Part model, mm, in its own coordinate system. Face numbers are marked on the shaded views. Give positions to 0.01 mm unless a question says otherwise; leave off trailing zeros. Write each loop counter-clockwise with the first axis right and the second up, starting at its lowest first coordinate (ties: lowest second). Pieces come first, ordered by that corner, then holes. Notation, with made-up numbers: M 43,88 L 66,88 A30 cw 66,120 Z; hole C 55,-23 d6. An arc over 180 degrees is marked long. Use a Markdown table: item, result.
```python
from build123d import *

# Parameters (mm, degrees)
F2_R = 1.49999


# Not quite as in the source:
# - a fillet or chamfer is up to 0.001 mm smaller than in the source, because OpenCascade refuses the exact size


with BuildPart() as f1:
    # F0 (on Right) → F1 (revolve)
    with BuildSketch(Plane.YZ):
        Polygon((43, 3), (43, 0), (60, 0), (69.0046720892, 153), (73.5, 153), (73.5, 156), (71, 156), (71, 170), (67, 170), (57.1713709877, 3), (46, 3), (46, 6), (0, 6), (0, 3), align=None)
    revolve(axis=Axis((0, 0, 4.5), (0, 0, -1)))

    # F2 (radius 1.5 in the source; OpenCascade refuses exactly that, so slightly less here)
    f2_edges = [f1.edges().sort_by_distance(p)[0] for p in [
        (0, -43, 0),
        (0, -60, 0),
        (0, -43, 3),
    ]]
    fillet(f2_edges, radius=F2_R)


solid = f1.part
```
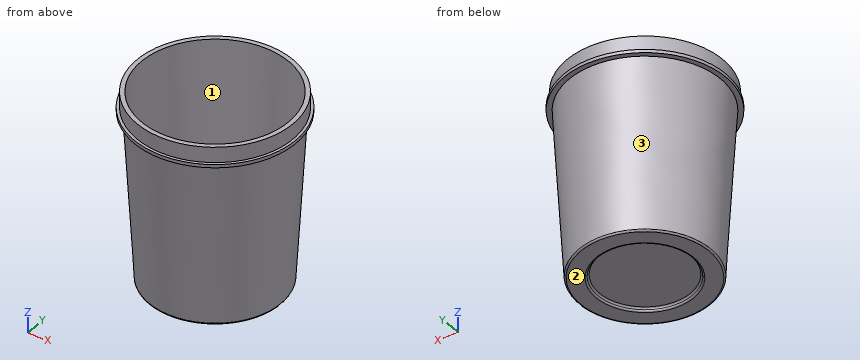
1. Cut at D-D, the plane z = 74. Give the cut face in (x, y), then the cut area to 3 significant figures.
Findings below:
| item | result |
|---|---|
| outline | C 0,0 d128.71; hole C 0,0 d122.7 |
| area | 1,190 mm2 |
2. Drop flat-ended pins along their axis: P1, Ø1.5, axis at x = -36.5, z = 97.5, coming from the +Y side; P2, Ø1, axis at x = -47.5, y = -4.5, coming from the +Z side; P3, Ø4, axis at x = -41.5, z = 137, coming from the +Y side. Give the stop position or say it passes through.
Findings below:
| item | result |
|---|---|
| P1 | y = 55.17 |
| P2 | z = 3 |
| P3 | y = 55.44 |
3. Drill centre lines: L1, parallel to X at y = 0, z = 1.55; L2, parallel to X at y = -33.5, z = 16; L3, parallel to Z at x = -11.5, y = -3. Where is each one in solid material? Low to high.
Findings below:
| item | result |
|---|---|
| L1 | -60.09 to -43, 43 to 60.09 |
| L2 | -50.91 to -47.27, 47.27 to 50.91 |
| L3 | 3 to 6 |
4. Cut at C-C, the plane z = 115. Give the cut face in (x, y), then the cut area to 3 significant figures.
Findings below:
| item | result |
|---|---|
| outline | C 0,0 d133.54; hole C 0,0 d127.53 |
| area | 1,230 mm2 |
5. Two-plate mould, pull along X, no slides. Class the marked faces 1, 2 and 3: released by +X, released by -X, zero draft, split by the parting line, or undercut.
Findings below:
| item | result |
|---|---|
| face 1 | undercut |
| face 2 | zero draft |
| face 3 | split by the parting line |
